from build123d import *

# Parameters (mm, degrees)
SKETCH_1_R           = 16
EXTRUDE_1_DEPTH      = 20
SKETCH_2_R           = 13
CUT_EXTRUDE_1_DEPTH  = 16
CUT_EXTRUDE_8_DEPTH  = 15
SKETCH_7_W           = 7.773458373
SKETCH_7_H           = 44.148318348
CUT_EXTRUDE_9_DEPTH  = 15
CUT_EXTRUDE_12_DEPTH = 15
CUT_EXTRUDE_14_DEPTH = 6


with BuildPart() as part:
    # 草图1 → 凸台-拉伸1 (new body)
    with BuildSketch(Plane(origin=(0, 0, 0), x_dir=(1, 0, 0), z_dir=(0, 1, 0))):
        with Locations(Location((0, 0, 0), (0, 0, 270))):
            Circle(SKETCH_1_R)
    extrude(amount=EXTRUDE_1_DEPTH)

    # 草图2 → 切除-拉伸1 (cut)
    with BuildSketch(Plane(origin=(0, 20, 0), x_dir=(1, 0, 0), z_dir=(0, 1, 0))):
        with Locations(Location((0, 0, 0), (0, 0, 270))):
            Circle(SKETCH_2_R)
    extrude(amount=-CUT_EXTRUDE_1_DEPTH, mode=Mode.SUBTRACT)

    # Sketch 3D_1 → 切除-拉伸8 (cut)
    with BuildSketch(Plane(origin=(-21.115525012, 20, -4.47842686), x_dir=(0.9837828296095457, 0, 0.17936372031555256), z_dir=(0, -1, 0))):
        Polygon((0, 0), (42.521972379, -7.752624798), (43.935434359, 0), (1.41346198, 7.752624798), align=None)
    extrude(amount=CUT_EXTRUDE_8_DEPTH, mode=Mode.SUBTRACT)

    # 草图7 → 切除-拉伸9 (cut)
    with BuildSketch(Plane(origin=(0, 20, 0), x_dir=(1, 0, 0), z_dir=(0, 1, 0))):
        with Locations((0.764910482, -0.180026065)):
            Rectangle(SKETCH_7_W, SKETCH_7_H)
    extrude(amount=-CUT_EXTRUDE_9_DEPTH, mode=Mode.SUBTRACT)

    # 草图8 → 切除-拉伸12 (cut)
    with BuildSketch(Plane(origin=(0, 20, 0), x_dir=(1, 0, 0), z_dir=(0, 1, 0))):
        Polygon((-0.220684434, -4.025865965), (-5.305815048, 1.059264649), (-20.221668569, -11.283691061), (-18.774175203, -19.378987698), align=None)
        Polygon((-12.618321187, 18.401718398), (-17.471521644, 13.224971244), (-5.305815048, 1.059264649), (-0.097842246, 5.368892492), align=None)
        with BuildLine():
            Line((9.217986526, 13.07779509), (6.801952348, 11.078512728))
            ThreePointArc((6.801952348, 11.078512728), (9.592762697, 8.773762239), (11.63996381, 5.788889574))
            Line((11.63996381, 5.788889574), (14.001568463, 7.743131187))
            ThreePointArc((14.001568463, 7.743131187), (11.912245515, 10.681685578), (9.217986526, 13.07779509))
        make_face()
        Polygon((4.875918089, 0.191602323), (-0.220684434, -4.025865965), (13.346301255, -17.592851655), (19.008368455, -14.519158032), align=None)
    extrude(amount=-CUT_EXTRUDE_12_DEPTH, mode=Mode.SUBTRACT)

    # Sketch 3D_2 → 切除-拉伸14 (cut)
    with BuildSketch(Plane(origin=(17.993102369, 20, -18.234682019), x_dir=(-0.7299619657231169, 0, 0.6834877677015465), z_dir=(0, -1, 0))):
        Polygon((0, 0), (27.649733988, 25.889369376), (51.890815184, 0), (24.241081197, -25.889369376), align=None)
    extrude(amount=CUT_EXTRUDE_14_DEPTH, mode=Mode.SUBTRACT)


solid = part.part
Can you work these out from the model? Positions are in its coordinate system, mm. A direction names the side the tool comes from. Give positions to 0.01 mm unless a question says otherwise; leave off trailing zeros. Loops run counter-clockwise (first coordinate to the right, second up) from the corner with the lowest first, then second, coordinate; pieces in that order, holes last. Notation, with made-up numbers: (-20, 61.25) -> (33, 61.25) arc R17 ccw to (33, 75.25) -> close; hole circle Ø8 at (30, 28.25). An arc over 180 degrees is marked (long way). Return JSON: item names as keys, results as strings.
Q1. I want a section at D-D, the plane y = 1. List the corners of the cut face in (x, z) for me, then the cut area to 3 significant figures.
Checks:
{"outline": "circle Ø32 at (0, 0)", "area": "804 mm2"}
Q2. We'd pull the mould along X, two halves only. Please class faces 1 (the face through (6, 14, -13)), 2 (the face through (1, 5, -15)): released by +X, released by -X, zero draft, split by the parting line, or undercut.
Checks:
{"face 1": "zero draft", "face 2": "undercut"}
Q3. I want a section at A-A, the plane y = 12.25. Count the separate pieces of the cut face and the enclosed holes in it, then the cut area to 3 significant figures.
Checks:
{"separate pieces": "8", "enclosed holes": "0", "area": "94.4 mm2"}
Q4. On a 3-axis mill with a long thin cutter (end or side, diameter ignored), from which of +Z, -Z, +X, -X, +Y, -Y can I reach the whole of each face in a straight line? I mean faces 3 (the face through (-12.167, 9.563, -7.92)), 4 (the face through (14, 5, 0)), 5 (the face through (0, 4, 0)), 6 (the face through (-13.347, 9.563, 5.595)), 7 (the face through (4.652, 10, 14)). Say none if no direction works.
Checks:
{"face 3": "-Z, +Y", "face 4": "+X, -X, +Y", "face 5": "+Y", "face 6": "+Z, +Y", "face 7": "+Z, -Z, +Y"}
Q5. For pin 1 Ø3.5 at (y, z) = (10.5, -14.5) entering from +X; pin 2 Ø0.9 at (y, z) = (9, 13.5) entering from +X; pin 3 Ø1 at (y, z) = (9.5, 14) entering from -X, each with a flat end and sliding along its axis, tell me the tip position at first contact or that it passes through.
Checks:
{"pin 1": "stops at x = 9.22", "pin 2": "stops at x = 8.99", "pin 3": "stops at x = -8.59"}
Q6. I want a section at B-B, the plane x = 0. List the corners of the cut face in (y, z) for me, then the cut area to 3 significant figures.
Checks:
{"outline": "(0, -16) -> (5, -16) -> (5, -13) -> (4, -13) -> (4, 13) -> (5, 13) -> (5, 16) -> (0, 16) -> close", "area": "134 mm2"}
Q7. I need wall thicknesses on probe 1 along Y at (x, z) = (10.5, 5); probe 2 along Y at (x, z) = (-8, -10.5); probe 3 along Z at (x, y) = (-7, 7.75). Which ranges of each line are inside material? Lowest first, please.
Checks:
{"probe 1": "y = 0 to 4", "probe 2": "y = 0 to 5", "probe 3": "z = -14.39 to -12.55, 10.95 to 14.39"}
Q8. I want a section at C-C, the plane z = 2. List the corners of the cut face in (x, y) for me, then the cut area to 3 significant figures.
Checks:
{"outline": "(-15.87, 0) -> (15.87, 0) -> (15.87, 5) -> (12.85, 5) -> (12.85, 4) -> (-12.85, 4) -> (-12.85, 5) -> (-15.87, 5) -> close", "area": "133 mm2"}
